Geometry check sheet. Reference: the model listing, model coordinates, mm. Face numbers are marked on the shaded views. A direction names the side the tool comes from. Round coordinates to 2 decimals unless told otherwise and drop trailing zeros. Order: outer loops, then holes, each group sorted by start corner. A loop starts at its lowest first (then second) coordinate and runs counter-clockwise, first axis right, second up. Notation, with made-up numbers: (32, 42) - (39, 42) arc R26 ccw to (39, 69) - close; hole circle Ø5 at (56.5, -2.75). An arc over 180 degrees is marked (long way). Return JSON: item names as keys, results as strings. Group by question number.
Q1. Draft check along Z on the marked faces 4, 5, 6 and 7. Enter one of: pulls with the +Z half, pulls with the -Z half, needs draft (parallel to the pull), parting line crosses it, or undercut.
Q2. Material ranges on line 1 along X through (y, z) = (6.5, -5.5); line 2 along Y through (x, z) = (0.5, -3.75); line 3 along X through (y, z) = (5.75, -3.5), recorded low to high.
Q3. Sectioned sample at D-D, the plane y = 2.5. Record the cut outline in (x, z).
Q4. Sectioned sample at B-B, the plane x = 0.75. Record the cut outline in (y, z), then the cut area to 3 significant figures.
Q5. Tool access check on the marked faces 1, 2 and 3. Record the directions out of +Z, -Z, +X, -X, +Y, -Y that give a thin tool (end or side, any length) a straight path to the whole face; none if there is none.
Q6. Sectioned sample at A-A, the plane y = 6. Record the cut outline in (x, z).
Q7. Sectioned sample at C-C, the plane z = -8.5. Record the cut outline in (x, y), then the cut area to 3 significant figures.
Q8. Gauge pin test, flat ends, axial feed: pin 1 Ø0.8 at (y, z) = (4, -1) entering from +X; pin 2 Ø4 at (x, y) = (0, 6) entering from +Z; pin 3 Ø3 at (x, y) = (5.5, 6.5) entering from +Z; pin 4 Ø4 at (x, z) = (3, -9) entering from -Y. Record the tip position at first contact, or that the pin passes through.
```python
from build123d import *

# Parameters (mm, degrees)
BOSS_EXTRUDE1_DEPTH = 5.207
CUT_EXTRUDE1_DEPTH  = 5.207
CUT_EXTRUDE2_DEPTH  = 5.207
FILLET1_R           = 0.4064
FILLET2_R           = 0.8128
BOSS_EXTRUDE2_DEPTH = 6.35


with BuildPart() as part:
    # Sketch1 → Boss-Extrude1 (new body)
    with BuildSketch(Plane(origin=(0, 0, 0), x_dir=(0, 0, -1), z_dir=(1, 0, 0))):
        Polygon((-0.2032, 0), (-0.2032, 5.3848), (10.3632, 5.3848), (10.3632, 0), (9.9568, 0), (9.9568, 4.9784), (0.2032, 4.9784), (0.2032, 0), align=None)
    extrude(amount=BOSS_EXTRUDE1_DEPTH)

    # Sketch2 → Cut-Extrude1 (cut)
    with BuildSketch(Plane(origin=(0, 0, -10.3632), x_dir=(-1, 0, 0), z_dir=(0, 0, -1))):
        with BuildLine():
            Line((-1.3335, 2.278639677), (-1.3335, 3.81))
            Line((-1.3335, 3.81), (0, 3.81))
            Line((0, 3.81), (0, -0.271412918))
            Line((0, -0.271412918), (-5.207, -0.271412918))
            Line((-5.207, -0.271412918), (-5.207, 3.81))
            Line((-5.207, 3.81), (-3.8735, 3.81))
            Line((-3.8735, 3.81), (-3.8735, 2.278639677))
            Line((-3.8735, 2.278639677), (-3.196682612, 0.419099186))
            ThreePointArc((-3.196682612, 0.419099186), (-2.6035, 0.003748249), (-2.010317388, 0.419099186))
            Line((-2.010317388, 0.419099186), (-1.3335, 2.278639677))
        make_face()
    extrude(amount=-CUT_EXTRUDE1_DEPTH, mode=Mode.SUBTRACT)

    # Sketch4 → Cut-Extrude2 (cut)
    with BuildSketch(Plane.XY.offset(0.2032)):
        with BuildLine():
            Line((0, 3.81), (0, -0.293581738))
            Line((0, -0.293581738), (5.207, -0.293581738))
            Line((5.207, -0.293581738), (5.207, 3.81))
            Line((5.207, 3.81), (3.3909, 3.81))
            Line((3.3909, 3.81), (3.3909, 2.362163271))
            Line((3.3909, 2.362163271), (2.849955114, 0.192551839))
            ThreePointArc((2.849955114, 0.192551839), (2.6035, 0), (2.357044886, 0.192551839))
            Line((2.357044886, 0.192551839), (1.8161, 2.362163271))
            Line((1.8161, 2.362163271), (1.8161, 3.81))
            Line((1.8161, 3.81), (0, 3.81))
        make_face()
    extrude(amount=-CUT_EXTRUDE2_DEPTH, mode=Mode.SUBTRACT)

    # Fillet1
    fillet1_edges = [part.edges().sort_by_distance(p)[0] for p in [
        (2.6035, 4.9784, -9.9568),
        (2.6035, 4.9784, -0.2032),
    ]]
    fillet(fillet1_edges, radius=FILLET1_R)

    # Fillet2
    fillet2_edges = [part.edges().sort_by_distance(p)[0] for p in [
        (2.6035, 5.3848, 0.2032),
        (2.6035, 5.3848, -10.3632),
    ]]
    fillet(fillet2_edges, radius=FILLET2_R)

    # Sketch5 → Boss-Extrude2 (add)
    with BuildSketch(Plane(origin=(0, 0, -9.5504), x_dir=(-1, 0, 0), z_dir=(0, 0, -1))):
        with BuildLine():
            Line((1.0922, 5.7912), (1.0922, 6.515909549))
            ThreePointArc((1.0922, 6.515909549), (-0.634040977, 7.863002154), (-1.9939, 6.1468))
            Line((-1.9939, 6.1468), (-1.584040966, 6.1468))
            ThreePointArc((-1.584040966, 6.1468), (-0.620193607, 7.454832725), (0.6858, 6.488224201))
            Line((0.6858, 6.488224201), (0.6858, 5.7912))
            ThreePointArc((0.6858, 5.7912), (0.566768196, 5.503831804), (0.2794, 5.3848))
            Line((0.2794, 5.3848), (0, 5.3848))
            Line((0, 5.3848), (0, 4.9784))
            Line((0, 4.9784), (0.2794, 4.9784))
            ThreePointArc((0.2794, 4.9784), (0.854136392, 5.216463608), (1.0922, 5.7912))
        make_face()
        with BuildLine():
            Line((-5.207, 4.9784), (-5.207, 5.3848))
            Line((-5.207, 5.3848), (-5.4864, 5.3848))
            ThreePointArc((-5.4864, 5.3848), (-5.773768196, 5.503831804), (-5.8928, 5.7912))
            Line((-5.8928, 5.7912), (-5.8928, 6.488224201))
            ThreePointArc((-5.8928, 6.488224201), (-4.586806393, 7.454832725), (-3.622959034, 6.1468))
            Line((-3.622959034, 6.1468), (-3.2131, 6.1468))
            ThreePointArc((-3.2131, 6.1468), (-4.572959023, 7.863002154), (-6.2992, 6.515909549))
            Line((-6.2992, 6.515909549), (-6.2992, 5.7912))
            ThreePointArc((-6.2992, 5.7912), (-6.061136392, 5.216463608), (-5.4864, 4.9784))
            Line((-5.4864, 4.9784), (-5.207, 4.9784))
        make_face()
    extrude(amount=-BOSS_EXTRUDE2_DEPTH)


solid = part.part
```
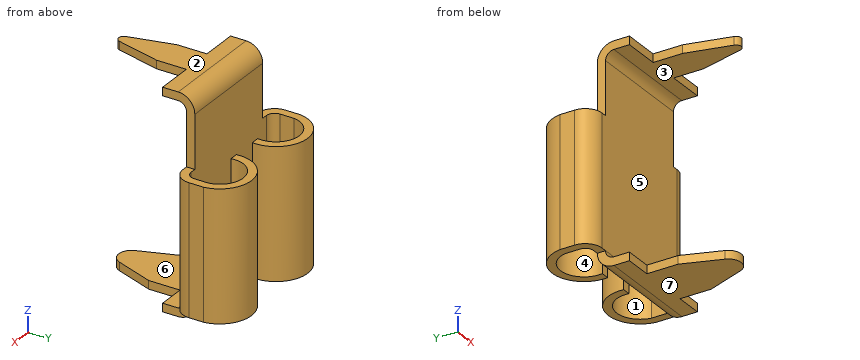
Reply:
{
 "1": {"face 4": "needs draft", "face 5": "undercut", "face 6": "undercut", "face 7": "pulls with the -Z half"},
 "2": {"line 1": "-1.09 to -0.68, 1.58 to 1.99, 3.21 to 3.62, 5.89 to 6.3", "line 2": "4.98 to 5.38, 7.47 to 7.87", "line 3": "-1.09 to -0.68, 5.89 to 6.3"},
 "3": {"outline": "(1.33, -10.36) - (3.87, -10.36) - (3.87, -9.96) - (1.33, -9.96) - close; (1.82, -0.2) - (3.39, -0.2) - (3.39, 0.2) - (1.82, 0.2) - close"},
 "4": {"outline": "(3.81, -10.36) - (4.57, -10.36) arc R0.81 ccw to (5.38, -9.55) - (5.38, -0.61) arc R0.81 ccw to (4.57, 0.2) - (3.81, 0.2) - (3.81, -0.2) - (4.57, -0.2) arc R0.41 cw to (4.98, -0.61) - (4.98, -9.55) arc R0.41 cw to (4.57, -9.96) - (3.81, -9.96) - close; (7.43, -9.55) - (7.84, -9.55) - (7.84, -3.2) - (7.43, -3.2) - close", "area": "7.68 mm^2"},
 "5": {"face 1": "+Z, -Z", "face 2": "+Z, +X, -X, +Y, -Y", "face 3": "+X, -X, -Y"},
 "6": {"outline": "(-1.09, -9.55) - (-0.69, -9.55) - (-0.69, -3.2) - (-1.09, -3.2) - close; (5.89, -9.55) - (6.3, -9.55) - (6.3, -3.2) - (5.89, -3.2) - close"},
 "7": {"outline": "(-1.09, 5.79) arc R0.81 ccw to (-0.28, 4.98) - (5.49, 4.98) arc R0.81 ccw to (6.3, 5.79) - (6.3, 6.52) arc R1.55 ccw to (3.21, 6.15) - (3.62, 6.15) arc R1.15 cw to (5.89, 6.49) - (5.89, 5.79) arc R0.41 cw to (5.49, 5.38) - (-0.28, 5.38) arc R0.41 cw to (-0.69, 5.79) - (-0.69, 6.49) arc R1.15 cw to (1.58, 6.15) - (1.99, 6.15) arc R1.55 ccw to (-1.09, 6.52) - close", "area": "7.14 mm^2"},
 "8": {"pin 1": "through", "pin 2": "z = 0.2", "pin 3": "z = 0.06", "pin 4": "y = 0"}
}
